The figure shows three views and two pictorial views of one solid part (mm, origin at its lowest corner). Answer the questions. Give positions to 0.01 mm unless a question says otherwise; leave off trailing zeros. Loops run counter-clockwise (first coordinate to the right, second up) from the corner with the lowest first, then second, coordinate; pieces in that order, holes last. Notation, with made-up numbers: M -3,26.5 L 14,26.5 A22 cw 14,32.5 Z; hole C -9.75,60.25 d10. An arc over 180 degrees is marked long. Answer in a Markdown table with one row per item. Add a question column.
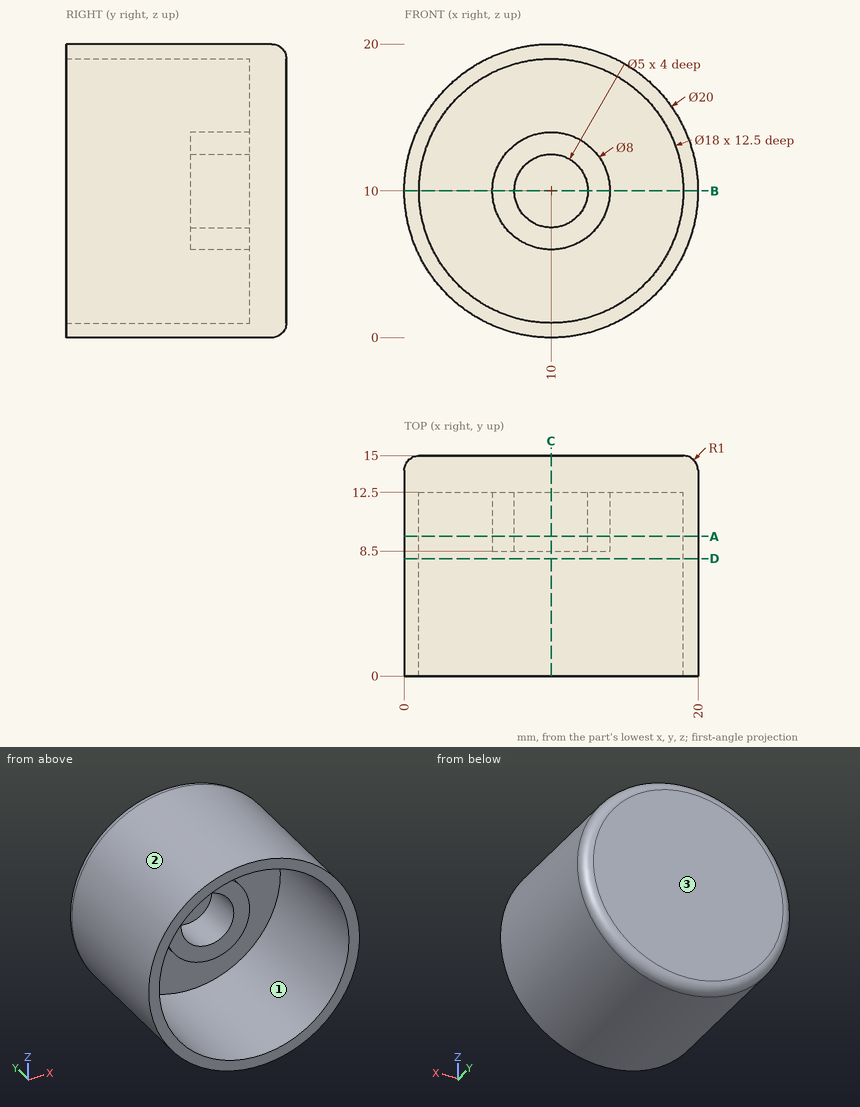
(1) Section A-A, the plane y = 9.5 is taken. Determine the outline of the cut face in (x, z), and give its area (3 significant figures).
(2) Section B-B, the plane z = 10 is taken. Determine the outline of the cut face in (x, y), and give its area (3 significant figures).
(3) The mould has two halves that part along Z. Classify the marked faces 1, 2 and 3: pulls with the +Z half, pulls with the -Z half, needs draft (parallel to the pull), parting line crosses it, or undercut.
(4) Section D-D, the plane y = 8 is taken. Determine the outline of the cut face in (x, z), and give its area (3 significant figures).
(5) Consider line 1 along X through (y, z) = (11.5, 10); line 2 along X through (y, z) = (7, 10). Determine where each line is inside the solid, lowest interval first. Write a range as from..to.
(6) Each of these flat-tipped pins is pushed along its axis until it touches: P1, Ø3, axis at x = 14, z = 7.5, coming from the -Y side; P2, Ø8, axis at x = 15, y = 3, coming from the +Z side; P3, Ø8, axis at x = 17.5, z = 15.5, coming from the +Y side; P4, Ø6, axis at x = 14, y = 6.5, coming from the -Z side. Where does it stop, or does it pass through?
(7) Section C-C, the plane x = 10 is taken. Determine the outline of the cut face in (y, z), and give its area (3 significant figures).
Numbers:
| question | item | result |
|---|---|---|
| 1 | outline | C 10,10 d20; C 10,10 d8; hole C 10,10 d18; hole C 10,10 d5 |
| 1 | area | 90.3 mm² |
| 2 | outline | M 0,0 L 1,0 L 1,12.5 L 6,12.5 L 6,8.5 L 7.5,8.5 L 7.5,12.5 L 12.5,12.5 L 12.5,8.5 L 14,8.5 L 14,12.5 L 19,12.5 L 19,0 L 20,0 L 20,14 A1 ccw 19,15 L 1,15 A1 ccw 0,14 Z |
| 2 | area | 86.6 mm² |
| 3 | face 1 | undercut |
| 3 | face 2 | parting line crosses it |
| 3 | face 3 | needs draft |
| 4 | outline | C 10,10 d20; hole C 10,10 d18 |
| 4 | area | 59.7 mm² |
| 5 | line 1 | x = 0..1, 6..7.5, 12.5..14, 19..20 |
| 5 | line 2 | x = 0..1, 19..20 |
| 6 | P1 | stops at y = 8.5 |
| 6 | P2 | stops at z = 19.95 |
| 6 | P3 | stops at y = 15 |
| 6 | P4 | stops at z = 0.05 |
| 7 | outline | M 0,0 L 14,0 A1 ccw 15,1 L 15,19 A1 ccw 14,20 L 0,20 L 0,19 L 12.5,19 L 12.5,14 L 8.5,14 L 8.5,12.5 L 12.5,12.5 L 12.5,7.5 L 8.5,7.5 L 8.5,6 L 12.5,6 L 12.5,1 L 0,1 Z |
| 7 | area | 86.6 mm² |
